from build123d import *

# Parameters (mm, degrees)
CYLINDER002_R     = 6
CYLINDER002_DEPTH = 8
CYLINDER001_R     = 3.1
CYLINDER001_DEPTH = 10
CYLINDER_R        = 10
CYLINDER_DEPTH    = 10
FILLET_R          = 1.8


with BuildPart() as cylinder002:
    # Cylinder002 → Cylinder002 (new body)
    with BuildSketch(Plane.XY.offset(2)):
        Circle(CYLINDER002_R)
    extrude(amount=CYLINDER002_DEPTH)


with BuildPart() as cylinder001:
    # Cylinder001 → Cylinder001 (new body)
    with BuildSketch(Plane.XY):
        Circle(CYLINDER001_R)
    extrude(amount=CYLINDER001_DEPTH)


with BuildPart() as fillet_body:
    # Cylinder → Cylinder (new body)
    with BuildSketch(Plane.XY):
        Circle(CYLINDER_R)
    extrude(amount=CYLINDER_DEPTH)

    # Cut: cut Cylinder001
    add(cylinder001.part, mode=Mode.SUBTRACT)

    # Cut001: cut Cylinder002
    add(cylinder002.part, mode=Mode.SUBTRACT)

    # Fillet
    fillet_edges = [fillet_body.edges().sort_by_distance(p)[0] for p in [
        (-10, 0, 10),
        (-6, 0, 10),
    ]]
    fillet(fillet_edges, radius=FILLET_R)


solid = fillet_body.part
Build history of the part. All positions in model axes, mm. A direction names the side the tool comes from. Round coordinates to 2 decimals unless told otherwise and drop trailing zeros. Write each loop counter-clockwise with the first axis right and the second up, starting at its lowest first coordinate (ties: lowest second). Pieces come first, ordered by that corner, then holes. Notation, with made-up numbers: M 16,0 L 44,0 A28 cw 44,29 Z; hole C 28.5,80 d6. An arc over 180 degrees is marked long. Answer as a JSON object with one key per item and string values. Group by question number.
(1) Which spindle directions (+Z, -Z, +X, -X, +Y, -Y) get a long thin tool onto all of the face, cutting with end or side? Do faces 4 (the flat face through (8, 0, 10)), 5 (the flat face through (3, -3, 2)). Say none if no direction does.
(2) Mould opens along Y. For faces 1 (the flat face through (-2.4, 2.4, 0)), 2 (the cylindrical face through (-2.17, -9.76, 4.04)), 3 (the cylindrical face through (-6, 0, 5)) say: pulls with the +Y half, pulls with the -Y half, needs draft (parallel to the pull), parting line crosses it, or undercut.
(3) Flat gauge pins, fed straight in: pin 1 (6 mm diameter, centred on x = 5, z = 7.5, fed in from +Y); pin 2 (6 mm diameter, centred on x = 1.5, y = 1.5, fed in from +Z); pin 3 (1 mm diameter, centred on x = -3.5, z = 2.5, fed in from -Y). Where does each tip first touch, or does it go through?
(4) Cut at A-A (y = 0). Give the cut face in (x, z).
(5) Drill centre lines: L1, parallel to Y at x = 0, z = 0.7; L2, parallel to X at y = -6.25, z = 2.25; L3, parallel to Z at x = -3, y = -3.5. Where is each one in solid material? Low to high.
(6) Cut at C-C (z = 7). Give the cut face in (x, y).
Responses:
{
 "1": {"face 4": "+Z, +X, -X, +Y, -Y", "face 5": "+Z"},
 "2": {"face 1": "needs draft", "face 2": "parting line crosses it", "face 3": "undercut"},
 "3": {"pin 1": "stops at y = 9.8", "pin 2": "stops at z = 2", "pin 3": "stops at y = -9.54"},
 "4": {"outline": "M -10,0 L -3.1,0 L -3.1,2 L -6,2 L -6,8.2 A1.8 ccw -7.8,10 L -8.2,10 A1.8 ccw -10,8.2 Z; M 3.1,0 L 10,0 L 10,8.2 A1.8 ccw 8.2,10 L 7.8,10 A1.8 ccw 6,8.2 L 6,2 L 3.1,2 Z"},
 "5": {"L1": "y = -10 to -3.1, 3.1 to 10", "L2": "x = -7.81 to 7.81", "L3": "z = 0 to 2"},
 "6": {"outline": "C 0,0 d20; hole C 0,0 d12"}
}
